Check sheet for the modelled part. Datum: model origin and axes. Units: mm. Give positions to 0.01 mm unless a question says otherwise; leave off trailing zeros. Order: outer loops, then holes, each group sorted by start corner. A loop starts at its lowest first (then second) coordinate and runs counter-clockwise, first axis right, second up.
```python
from build123d import *

# Parameters (mm, degrees)
SKETCH1_R           = 3
SKETCH1_R_2         = 4.5
SKETCH1_R_3         = 1.6
BOSS_EXTRUDE3_DEPTH = 1.6


with BuildPart() as part:
    # Sketch1 → Boss-Extrude3 (new body)
    with BuildSketch(Plane.XY):
        with BuildLine():
            Line((12.073070054, 14.639688463), (24.958502044, 12.880515151))
            ThreePointArc((24.958502044, 12.880515151), (36.2, 0), (24.958502044, -12.880515151))
            Line((24.958502044, -12.880515151), (12.073070054, -14.639688463))
            ThreePointArc((12.073070054, -14.639688463), (11.870633815, -14.660360595), (11.66726189, -14.66726189))
            Line((11.66726189, -14.66726189), (0, -14.66726189))
            ThreePointArc((0, -14.66726189), (-0.888679088, -14.53261518), (-1.697586366, -14.140761542))
            Line((-1.697586366, -14.140761542), (-18.697586366, -2.473499652))
            ThreePointArc((-18.697586366, -2.473499652), (-19.891071988, -0.801063519), (-19.728500117, 1.247111507))
            Line((-19.728500117, 1.247111507), (-14.395762007, 12.914373397))
            ThreePointArc((-14.395762007, 12.914373397), (-13.288783625, 14.191279968), (-11.66726189, 14.66726189))
            Line((-11.66726189, 14.66726189), (11.66726189, 14.66726189))
            ThreePointArc((11.66726189, 14.66726189), (11.870633815, 14.660360595), (12.073070054, 14.639688463))
        make_face()
        Circle(SKETCH1_R, mode=Mode.SUBTRACT)
        with Locations((23.2, 0)):
            Circle(SKETCH1_R_2, mode=Mode.SUBTRACT)
        with Locations((8.6, 0)):
            Circle(SKETCH1_R, mode=Mode.SUBTRACT)
        with Locations((-17, 0)):
            Circle(SKETCH1_R_3, mode=Mode.SUBTRACT)
        with Locations((0, -11.66726189)):
            Circle(SKETCH1_R_3, mode=Mode.SUBTRACT)
        with Locations((11.66726189, -11.66726189)):
            Circle(SKETCH1_R_3, mode=Mode.SUBTRACT)
        with Locations((-11.66726189, 11.66726189)):
            Circle(SKETCH1_R_3, mode=Mode.SUBTRACT)
        with Locations((0, 11.66726189)):
            Circle(SKETCH1_R_3, mode=Mode.SUBTRACT)
        with Locations((11.66726189, 11.66726189)):
            Circle(SKETCH1_R_3, mode=Mode.SUBTRACT)
    extrude(amount=BOSS_EXTRUDE3_DEPTH)


solid = part.part
```
Q1. Sectioned sample at C-C, the plane z = 0.35. Count the separate pieces of the cut face and the enclosed holes in it, plus the area to 3 significant figures.
Q2. Sectioned sample at D-D, the plane x = 23.2. Record the cut outline in (y, z).
Q3. Material ranges on line 1 (Y direction, x = 0, z = 1); line 2 (X direction, y = -0.75, z = 0.5); line 3 (X direction, y = -11, z = 0.55), recorded low to high.
Q4. Sectioned sample at B-B, the plane y = 0. Record the cut outline in (x, z).
Q5. Draft check along Y on faces 1 (the flat face through (18.43, 13.77, 0.79)), 2 (the cylindrical face through (12.527, 13.016, 0.789)), 3 (the cylindrical face through (-19.883, -0.829, 0.789)), 4 (the cylindrical face through (13.145, -12.28, 0.789)). Enter one of: pulls with the +Y half, pulls with the -Y half, needs draft (parallel to the pull), parting line crosses it, or undercut.
Q6. Sectioned sample at A-A, the plane x = 8.6. Record the cut outline in (y, z), plus the area to 3 significant figures.
Filled in:
1. separate pieces: 1
1. enclosed holes: 9
1. area: 1,180 mm2
2. outline: (-13.12, 0) - (-4.5, 0) - (-4.5, 1.6) - (-13.12, 1.6) - close; (4.5, 0) - (13.12, 0) - (13.12, 1.6) - (4.5, 1.6) - close
3. line 1: y = -14.67 to -13.27, -10.07 to -3, 3 to 10.07, 13.27 to 14.67
3. line 2: x = -19.9 to -18.41, -15.59 to -2.9, 2.9 to 5.7, 11.5 to 18.76, 27.64 to 36.18
3. line 3: x = -6.27 to -1.45, 1.45 to 10.21, 13.12 to 30.13
4. outline: (-20, 0) - (-18.6, 0) - (-18.6, 1.6) - (-20, 1.6) - close; (-15.4, 0) - (-3, 0) - (-3, 1.6) - (-15.4, 1.6) - close; (3, 0) - (5.6, 0) - (5.6, 1.6) - (3, 1.6) - close; (11.6, 0) - (18.7, 0) - (18.7, 1.6) - (11.6, 1.6) - close; (27.7, 0) - (36.2, 0) - (36.2, 1.6) - (27.7, 1.6) - close
5. face 1: pulls with the +Y half
5. face 2: undercut
5. face 3: parting line crosses it
5. face 4: undercut
6. outline: (-14.67, 0) - (-3, 0) - (-3, 1.6) - (-14.67, 1.6) - close; (3, 0) - (14.67, 0) - (14.67, 1.6) - (3, 1.6) - close
6. area: 37.3 mm2
